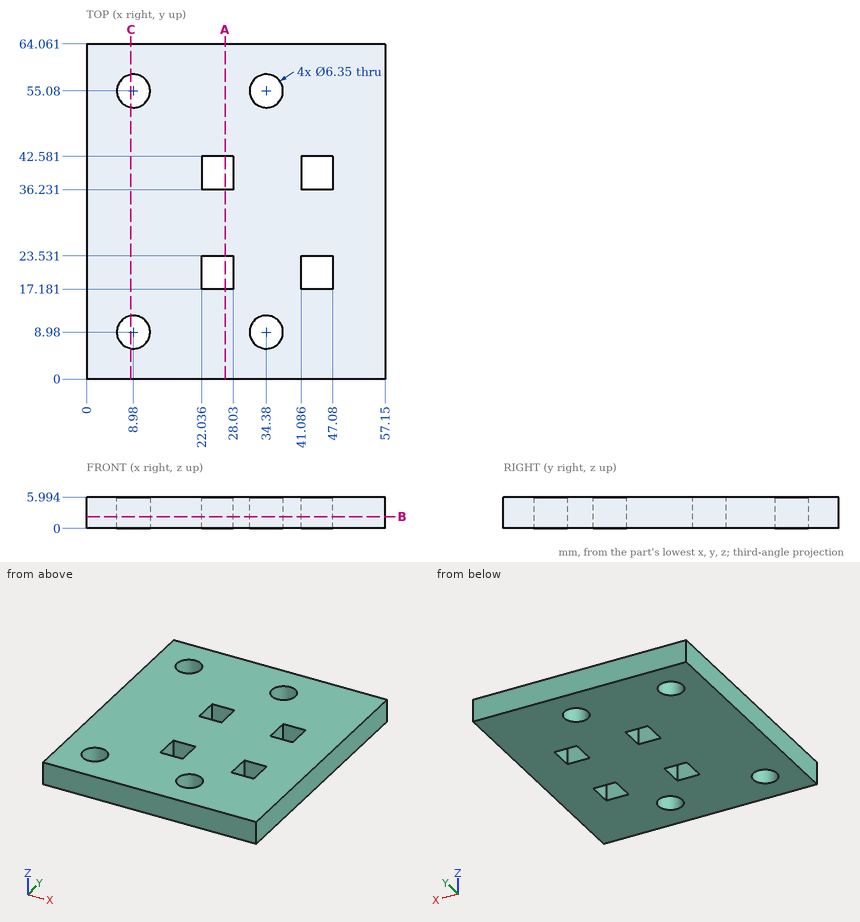
Print and shaded views of the part. All mm, measured from the part's lowest x, y and z. Give positions to 0.01 mm unless a question says otherwise; leave off trailing zeros. Loops run counter-clockwise (first coordinate to the right, second up) from the corner with the lowest first, then second, coordinate; pieces in that order, holes last. Notation, with made-up numbers: (-33, -35) -> (16, -35) arc R25 ccw to (16, -5) -> close; hole circle Ø3 at (10.5, 4). An arc over 180 degrees is marked (long way). Answer in a Markdown table with one row per item.
Item 1: Probe line 1 along Y through (x, z) = (46.5, 2.3); line 2 along Y through (x, z) = (9, 0.75) (1 decimal); line 3 along X through (y, z) = (56, 1.4). List the from-to ranges inside material, lowest first. Write a range as [from, to].
Findings below:
| item | result |
|---|---|
| line 1 | y = [0, 17.18], [23.53, 36.23], [42.58, 64.06] |
| line 2 | y = [0, 5.8], [12.2, 51.9], [58.3, 64.1] |
| line 3 | x = [0, 5.94], [12.02, 31.34], [37.42, 57.15] |
Item 2: Slice it at A-A on x = 26.5. Write the cut outline in (y, z) (1 decimal), plus the area to 3 significant figures.
Findings below:
| item | result |
|---|---|
| outline | (0, 0) -> (17.2, 0) -> (17.2, 6) -> (0, 6) -> close; (23.5, 0) -> (36.2, 0) -> (36.2, 6) -> (23.5, 6) -> close; (42.6, 0) -> (64.1, 0) -> (64.1, 6) -> (42.6, 6) -> close |
| area | 308 mm² |
Item 3: Slice it at C-C on x = 8.5. Write the cut outline in (y, z) (1 decimal).
Findings below:
| item | result |
|---|---|
| outline | (0, 0) -> (5.8, 0) -> (5.8, 6) -> (0, 6) -> close; (12.1, 0) -> (51.9, 0) -> (51.9, 6) -> (12.1, 6) -> close; (58.2, 0) -> (64.1, 0) -> (64.1, 6) -> (58.2, 6) -> close |
Item 4: Slice it at B-B on z = 2.25. Give the number of separate pieces and of enclosed holes in the cut face, plus the area to 3 significant figures.
Findings below:
| item | result |
|---|---|
| separate pieces | 1 |
| enclosed holes | 8 |
| area | 3,380 mm² |
